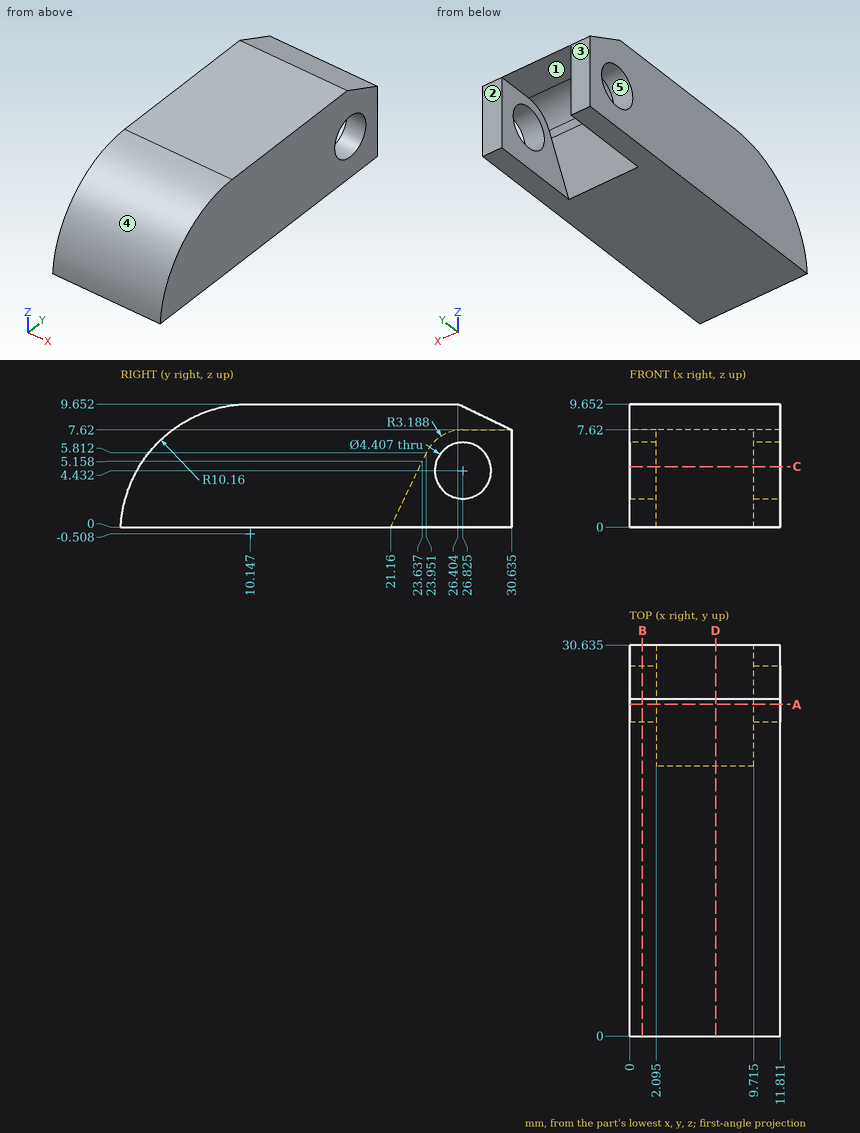
For this review, use the dimensioned drawing (mm, ordinates from the lowest corner) and the shaded views. A direction names the side the tool comes from. Round coordinates to 2 decimals unless told otherwise and drop trailing zeros. Write each loop counter-clockwise with the first axis right and the second up, starting at its lowest first coordinate (ties: lowest second). Pieces come first, ordered by that corner, then holes. Notation, with made-up numbers: M 6.5,13 L 36.5,13 A22 cw 36.5,50 Z; hole C 24.5,60 d11. An arc over 180 degrees is marked long. Answer as CSV lines item,"result". Start each with the question number.
Q1. Tool access review of the marked faces 1 and 2: name each direction out of +Z, -Z, +X, -X, +Y, -Y from which nothing blocks a thin tool from reaching the whole face with its end or side.
Q2. Consider section C-C, the plane z = 4.75. Give the boundary of the cut face in (x, y) (1 decimal).
Q3. The part is to be moulded in two halves that separate along Z. For the marked faces 3, 4 and 5, say which applies: +Z half, -Z half, draft (parallel to the pull), parting line (faces both ways), or undercut.
Q4. Consider section B-B, the plane x = 1. Give the boundary of the cut face in (y, z) (1 decimal).
Q5. Consider section A-A, the plane y = 26. Give the boundary of the cut face in (x, z) (1 decimal).
Q6. Clearance check with flat-ended pins moving along their axes: P1, Ø2.5, axis at y = 26.82, z = 4.43, coming from the +X side; P2, Ø3, axis at x = 7, y = 28.5, coming from the -Z side; P3, Ø3, axis at x = 6.5, y = 24.5, coming from the -Z side; P4, Ø5, axis at x = 4.5, z = 4, coming from the -Y side. State where each tip first meets the part, or that it passes through.
Q7. Consider section D-D, the plane x = 6.75. Give the boundary of the cut face in (y, z) (1 decimal), then the cut area to 3 significant figures.
Q8. Wall thickness on line 1 along X through (y, z) = (25, 6.25) (1 decimal); line 2 along Y through (x, z) = (1, 2.5) (1 decimal); line 3 along Y through (x, z) = (1.5, 3.5) (1 decimal): over which ranges is each line inside the solid? List them lowest first.
Result set:
1,face 1,"-Z, +Y"
1,face 2,"+Z, -Z, +X, -X, +Y"
2,outline,"M 0,1.5 L 11.8,1.5 L 11.8,24.6 L 9.7,24.6 L 9.7,23.4 L 2.1,23.4 L 2.1,24.6 L 0,24.6 Z; M 0,29 L 2.1,29 L 2.1,30.6 L 0,30.6 Z; M 9.7,29 L 11.8,29 L 11.8,30.6 L 9.7,30.6 Z"
3,face 3,"draft"
3,face 4,"+Z half"
3,face 5,"undercut"
4,outline,"M 0,0 L 30.6,0 L 30.6,7.6 L 26.4,9.7 L 10.1,9.7 A10.2 ccw Z; hole C 26.8,4.4 d4.4"
5,outline,"M 0,0 L 2.1,0 L 2.1,2.4 L 0,2.4 Z; M 0,6.5 L 2.1,6.5 L 2.1,7.5 L 9.7,7.5 L 9.7,6.5 L 11.8,6.5 L 11.8,9.7 L 0,9.7 Z; M 9.7,0 L 11.8,0 L 11.8,2.4 L 9.7,2.4 Z"
6,P1,"passes through"
6,P2,"stops at z = 7.62"
6,P3,"stops at z = 3.83"
6,P4,"stops at y = 0.19"
7,outline,"M 0,0 L 21.2,0 L 24,5.8 A3.2 cw 26.8,7.6 L 30.6,7.6 L 26.4,9.7 L 10.1,9.7 A10.2 ccw Z"
7,area,"212 mm²"
8,line 1,"x = 0 to 2.1, 9.7 to 11.8"
8,line 2,"y = 0.4 to 25.8, 27.9 to 30.6"
8,line 3,"y = 0.8 to 24.8, 28.8 to 30.6"
